Input: part model. Units: mm. Frame: model coordinates. Face numbers are marked on the shaded views. Coordinates: 2 decimals unless noted, no trailing zeros. Order: outer loops, then holes, each group sorted by start corner. A loop starts at its lowest first (then second) coordinate and runs counter-clockwise, first axis right, second up. Notation, with made-up numbers: (-7, 74.25) -> (19, 74.25) arc R33 cw to (19, 104.25) -> close; hole circle Ø10 at (2, 66.5). An arc over 180 degrees is marked (long way). Answer as CSV lines item,"result".
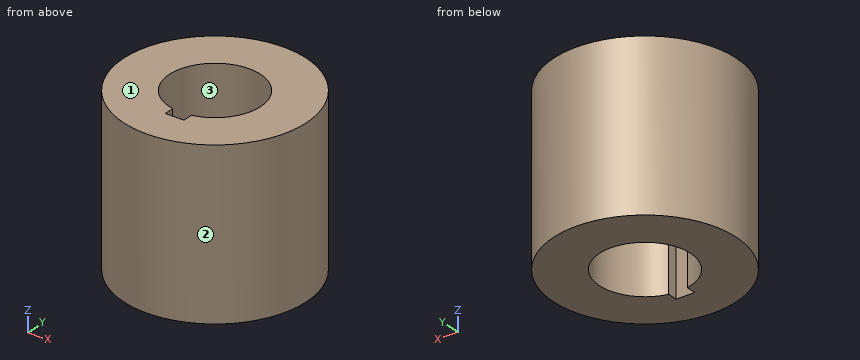
from build123d import *

# Parameters (mm, degrees)
F0_R     = 100
F1_DEPTH = 180
F2_R     = 50
F3_DEPTH = 180.001
F4_W     = 20.454546
F4_H     = 19.62437
F5_DEPTH = 180.001


with BuildPart() as f1:
    # F0 (on Top) → F1 (new body)
    with BuildSketch(Plane.XY):
        Circle(F0_R)
    extrude(amount=F1_DEPTH)

    # F2 (on face) → F3 (cut, through all)
    with BuildSketch(Plane.XY.offset(180)):
        Circle(F2_R)
    extrude(amount=-F3_DEPTH, mode=Mode.SUBTRACT)

    # F4 (on face) → F5 (cut, through all)
    with BuildSketch(Plane.XY.offset(180)):
        with Locations((0.227273, -50.187815)):
            Rectangle(F4_W, F4_H)
    extrude(amount=-F5_DEPTH, mode=Mode.SUBTRACT)


solid = f1.part
1. Contact query for flat-ended pins moving along their axis: pin 1 (4 mm diameter, centred on y = 69.5, z = 36.5, fed in from -X); pin 2 (8 mm diameter, centred on x = -50, z = 115.5, fed in from +Y); pin 3 (12 mm diameter, centred on y = -54.5, z = 73.5, fed in from -X). Output: stop coordinate, or through.
Findings:
pin 1,"stops at x = -73.78"
pin 2,"stops at y = 88.79"
pin 3,"stops at x = -87.45"
2. Ray query, line 1 along Y through (x, z) = (0, 116); line 2 along Y through (x, z) = (4, 98.5); line 3 along X through (y, z) = (35, 27). Return the intervals inside material, ascending.
Findings:
line 1,"y = -100 to -60, 50 to 100"
line 2,"y = -99.92 to -60, 49.84 to 99.92"
line 3,"x = -93.67 to -35.71, 35.71 to 93.67"
3. Cut plane A-A (x = 0). Return the cut outline in (y, z).
Findings:
outline,"(-100, 0) -> (-60, 0) -> (-60, 180) -> (-100, 180) -> close; (50, 0) -> (100, 0) -> (100, 180) -> (50, 180) -> close"
4. Mould query, pull axis X, two halves, no side actions, for the marked faces 1, 2 and 3. Classes: released by +X, released by -X, zero draft, split by the parting line, or undercut.
Findings:
face 1,"zero draft"
face 2,"split by the parting line"
face 3,"undercut"
5. Cut plane D-D (y = 83.5). Return the cut outline in (x, z) (3 decimals).
Findings:
outline,"(-55.025, 0) -> (55.025, 0) -> (55.025, 180) -> (-55.025, 180) -> close"
6. Cut plane C-C (y = 0). Return the cut outline in (x, z), plus the area to 3 significant figures.
Findings:
outline,"(-100, 0) -> (-50, 0) -> (-50, 180) -> (-100, 180) -> close; (50, 0) -> (100, 0) -> (100, 180) -> (50, 180) -> close"
area,"18,000 mm2"
7. Cut plane B-B (z = 120.5). Return the cut outline in (x, y), plus the area to 3 significant figures.
Findings:
outline,"circle Ø200 at (0, 0); hole (-10, -60) -> (10.45, -60) -> (10.45, -48.89) arc R50 ccw (long way) to (-10, -48.99) -> close"
area,"23,400 mm2"
